from build123d import *

# Parameters (mm, degrees)
BOSS_EXTRUDE1_DEPTH = 120
RIB2_REACH          = 80.102
SKETCH2_WALL_W      = 194.127281078
SKETCH2_WALL_H      = 5
RIB3_REACH          = 118.297
SKETCH3_WALL_W      = 270.649579746
SKETCH3_WALL_H      = 5
RIB4_REACH          = 118.297
SKETCH4_WALL_W      = 270.649579746
SKETCH4_WALL_H      = 5


with BuildPart() as part:
    # Sketch1 → Boss-Extrude1 (new body)
    with BuildSketch(Plane.XY):
        Polygon((0, 40), (0, 0), (30, 0), (30, 10), (10, 10), (10, 40), align=None)
    extrude(amount=BOSS_EXTRUDE1_DEPTH)

    # Sketch2 wall → Rib2 (add, up to next)
    with BuildSketch(Plane(origin=(19.879407162, 25, 60), x_dir=(0.550043320359, -0.835136124071, 0), z_dir=(0.835136124071, 0.550043320359, 0)), mode=Mode.PRIVATE) as rib2_sk1:
        Rectangle(SKETCH2_WALL_W, SKETCH2_WALL_H)
    rib2_tool1 = extrude(rib2_sk1.sketch, amount=-RIB2_REACH, mode=Mode.PRIVATE) - part.part
    add(rib2_tool1.solids().sort_by_distance((19.879407162, 25, 60))[0])

    # Sketch3 wall → Rib3 (add, up to next)
    with BuildSketch(Plane(origin=(20, 25, 105), x_dir=(0.554700196225, -0.832050294338, 0), z_dir=(0.832050294338, 0.554700196225, 0)), mode=Mode.PRIVATE) as rib3_sk1:
        Rectangle(SKETCH3_WALL_W, SKETCH3_WALL_H)
    rib3_tool1 = extrude(rib3_sk1.sketch, amount=-RIB3_REACH, mode=Mode.PRIVATE) - part.part
    add(rib3_tool1.solids().sort_by_distance((20, 25, 105))[0])

    # Sketch4 wall → Rib4 (add, up to next)
    with BuildSketch(Plane(origin=(20, 25, 15), x_dir=(0.554700196225, -0.832050294338, 0), z_dir=(0.832050294338, 0.554700196225, 0)), mode=Mode.PRIVATE) as rib4_sk1:
        Rectangle(SKETCH4_WALL_W, SKETCH4_WALL_H)
    rib4_tool1 = extrude(rib4_sk1.sketch, amount=-RIB4_REACH, mode=Mode.PRIVATE) - part.part
    add(rib4_tool1.solids().sort_by_distance((20, 25, 15))[0])


solid = part.part
Model file for the job. Use its own axes, mm. A direction names the side the tool comes from. Round coordinates to 2 decimals unless told otherwise and drop trailing zeros. Loops run counter-clockwise (first coordinate to the right, second up) from the corner with the lowest first, then second, coordinate; pieces in that order, holes last.
1. Band-saw the part on C-C, the plane y = 35.5. List the corners of the cut face in (x, z), and give its area (3 significant figures).
Check values:
outline: (0, 0) - (10, 0) - (10, 12.5) - (13, 12.5) - (13, 17.5) - (10, 17.5) - (10, 57.5) - (12.96, 57.5) - (12.96, 62.5) - (10, 62.5) - (10, 102.5) - (13, 102.5) - (13, 107.5) - (10, 107.5) - (10, 120) - (0, 120) - close
area: 1,240 mm2
2. Band-saw the part on B-B, the plane x = 21.25. List the corners of the cut face in (y, z) (3 decimals).
Check values:
outline: (0, 0) - (10, 0) - (10, 12.5) - (23.125, 12.5) - (23.125, 17.5) - (10, 17.5) - (10, 57.5) - (22.919, 57.5) - (22.919, 62.5) - (10, 62.5) - (10, 102.5) - (23.125, 102.5) - (23.125, 107.5) - (10, 107.5) - (10, 120) - (0, 120) - close
3. Drop flat-ended pins along their axis: P1, Ø12, axis at x = 24.5, z = 31.5, coming from the +Y side; P2, Ø6, axis at y = 25, z = 4, coming from the +X side; P3, Ø10, axis at x = 21, y = 19, coming from the -Z side. Give the stop position or say it passes through.
Check values:
P1: stops at y = 10
P2: stops at x = 10
P3: stops at z = 12.5
4. Band-saw the part on D-D, the plane z = 61. List the corners of the cut face in (x, y), and give its area (3 significant figures).
Check values:
outline: (0, 0) - (30, 0) - (30, 10) - (29.76, 10) - (10, 40) - (0, 40) - close
area: 896 mm2
5. Mould opens along Z. For faces 1 (the flat face through (17, 18, 62.5)), 2 (the flat face through (10, 25, 6)), 3 (the flat face through (18, 19, 107.5)) say: +Z half, -Z half, draft (parallel to the pull), parting line (faces both ways), or undercut.
Check values:
face 1: undercut
face 2: draft
face 3: +Z half
6. Tool access for faces 4 (the flat face through (20, 10, 50)), 5 (the flat face through (18, 19, 12.5)), 6 (the flat face through (20, 10, 114)): list every direction of +Z, -Z, +X, -X, +Y, -Y with a clear straight run to the whole face (end or side of a thin tool).
Check values:
face 4: +X, +Y
face 5: -Z, +X, +Y
face 6: +Z, +X, +Y
7. Wall check: probe 1 along Z at (x, y) = (19, 12); probe 2 along Y at (x, z) = (17.5, 85). Give the ranges that are in metal, low to high.
Check values:
probe 1: z = 12.5 to 17.5, 57.5 to 62.5, 102.5 to 107.5
probe 2: y = 0 to 10
8. Band-saw the part on A-A, the plane z = 75.5. List the corners of the cut face in (x, y), and give its area (3 significant figures).
Check values:
outline: (0, 0) - (30, 0) - (30, 10) - (10, 10) - (10, 40) - (0, 40) - close
area: 600 mm2
